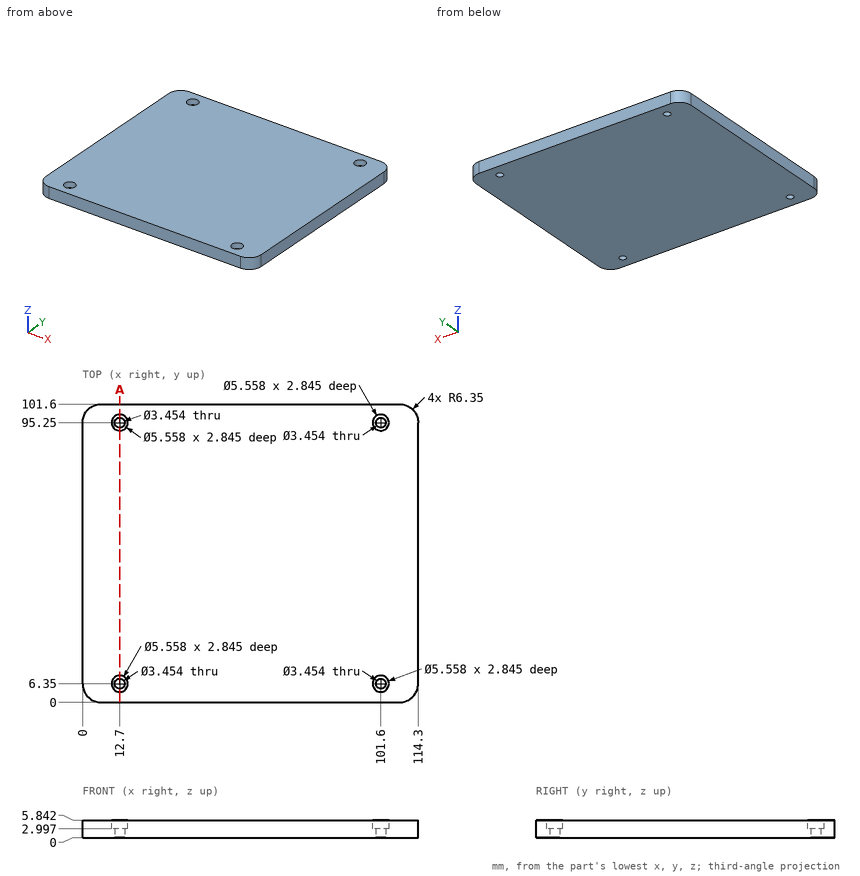
Part print with two shaded views. Sizes in mm from the minimum x, y, z corner. Coordinates: 2 decimals unless noted, no trailing zeros. Loops run counter-clockwise (first coordinate to the right, second up) from the corner with the lowest first, then second, coordinate; pieces in that order, holes last. Notation, with made-up numbers: (-7, -11.75) - (6, -11.75) arc R18 cw to (6, 17.25) - close; hole circle Ø9 at (60.25, -37). An arc over 180 degrees is marked (long way). Write each question's results on one line, items separated by ' | '. Start each with the question number.
Q1. Probe line 1 along Y through (x, z) = (101.6, 1.3); line 2 along X through (y, z) = (95.25, 1.5); line 3 along Y through (x, z) = (101.6, 4.9). List the from-to ranges inside material, lowest first.
Q2. Drop flat-ended pins along their axis: pin 1 Ø5 at (x, y) = (101.6, 95.25) entering from +Z; pin 2 Ø1.7 at (x, y) = (101, 95) entering from +Z. Give the stop position or say it passes through.
Q3. Slice it at A-A on x = 12.7. Give the cut face in (y, z).
Answer:
1) line 1: y = 0 to 4.62, 8.08 to 93.52, 96.98 to 101.6 | line 2: x = 0 to 10.97, 14.43 to 99.87, 103.33 to 114.3 | line 3: y = 0 to 3.57, 9.13 to 92.47, 98.03 to 101.6
2) pin 1: stops at z = 3 | pin 2: passes through
3) outline: (0, 0) - (4.62, 0) - (4.62, 3) - (3.57, 3) - (3.57, 5.84) - (0, 5.84) - close; (8.08, 0) - (93.52, 0) - (93.52, 3) - (92.47, 3) - (92.47, 5.84) - (9.13, 5.84) - (9.13, 3) - (8.08, 3) - close; (96.98, 0) - (101.6, 0) - (101.6, 5.84) - (98.03, 5.84) - (98.03, 3) - (96.98, 3) - close
